```python
from build123d import *

# Parameters (mm, degrees)
F0_W     = 50.8
F0_H     = 50.8
F1_DEPTH = 304.8
F2_R     = 5.08
F3_W     = 6.35
F3_H     = 38.1
F4_DEPTH = 304.8
F5_W     = 50.8
F5_H     = 50.8
F6_DEPTH = 304.8
F7_R     = 5.08


with BuildPart() as f1:
    # F0 (on Top) → F1 (new body)
    with BuildSketch(Plane.XY):
        with Locations((25.4, -25.4)):
            Rectangle(F0_W, F0_H)
    extrude(amount=F1_DEPTH)

    # F2
    f2_edges = [f1.edges().sort_by_distance(p)[0] for p in [
        (0, -50.8, 152.4),
        (50.8, -50.8, 152.4),
        (50.8, 0, 152.4),
        (0, 0, 152.4),
    ]]
    fillet(f2_edges, radius=F2_R)

    # F3 (on Top) → F4 (join)
    with BuildSketch(Plane.XY):
        with Locations((-3.175, -25.4)):
            Rectangle(F3_W, F3_H)
    extrude(amount=F4_DEPTH)

    # F5 (on Top) → F6 (join)
    with BuildSketch(Plane.XY):
        with Locations((-31.75, -25.4)):
            Rectangle(F5_W, F5_H)
    extrude(amount=F6_DEPTH)

    # F7
    f7_edges = [f1.edges().sort_by_distance(p)[0] for p in [
        (-57.15, -50.8, 152.4),
        (-6.35, -50.8, 152.4),
        (-57.15, 0, 152.4),
        (-6.35, 0, 152.4),
    ]]
    fillet(f7_edges, radius=F7_R)


solid = f1.part
```
For this review, take the finished solid that the model builds, in its own axes (mm). A direction names the side the tool comes from. Round coordinates to 2 decimals unless told otherwise and drop trailing zeros. Write each loop counter-clockwise with the first axis right and the second up, starting at its lowest first coordinate (ties: lowest second). Pieces come first, ordered by that corner, then holes.
1) Take a section at A-A on z = 144.5. Give the boundary of the cut face in (x, y), then the cut area to 3 significant figures.
Answer below:
outline: (-57.15, -45.72) arc R5.08 ccw to (-52.07, -50.8) - (-11.43, -50.8) arc R5.08 ccw to (-6.35, -45.72) - (-6.35, -44.45) - (0, -44.45) - (0, -45.72) arc R5.08 ccw to (5.08, -50.8) - (45.72, -50.8) arc R5.08 ccw to (50.8, -45.72) - (50.8, -5.08) arc R5.08 ccw to (45.72, 0) - (5.08, 0) arc R5.08 ccw to (0, -5.08) - (0, -6.35) - (-6.35, -6.35) - (-6.35, -5.08) arc R5.08 ccw to (-11.43, 0) - (-52.07, 0) arc R5.08 ccw to (-57.15, -5.08) - close
area: 5,360 mm2
2) Insertion check: pin 1 Ø3 at (x, z) = (-2, 100.5) entering from -Y; pin 2 Ø5 at (x, z) = (-3, 131) entering from +Y. Each pin has a flat end and moves straight along its axis. Give the tip position at first contact, or say it passes through.
Answer below:
pin 1: stops at y = -44.45
pin 2: stops at y = -6.35
3) For line 1 along X through (y, z) = (-44.5, 48.5), list the stretches that pass through material, from the lowest coordinate up.
Answer below:
line 1: x = -57.15 to -6.35, 0 to 50.8
4) Machinability: for faces 4 (the face through (1.449, -49.272, 154.534)), 5 (the face through (-7.878, -1.449, 154.534)), 6 (the face through (-32, 0, 150)), which of the approach directions +Z, -Z, +X, -X, +Y, -Y give a long, thin tool a straight path to every point of the face, cutting with its end or side? Answer none if there is none.
Answer below:
face 4: +Z, -Z, -Y
face 5: +Z, -Z, +Y
face 6: +Z, -Z, +X, -X, +Y
5) Mouldability with a two-part tool opening along X and no side actions: class faces 1 (the face through (49.272, -49.351, 154.534)), 2 (the face through (-3, -44.45, 150)), 3 (the face through (-4, -25, 304.8)) as +X half, -X half, draft (parallel to the pull), parting line (faces both ways), or undercut.
Answer below:
face 1: +X half
face 2: undercut
face 3: draft
